Geometry check sheet. Reference: the model listing, model coordinates, mm. Face numbers are marked on the shaded views. A direction names the side the tool comes from. Coordinates: 2 decimals unless noted, no trailing zeros. Answer in a Markdown table with one row per item. Add a question column.
1. Mould release check, pull along Y, two halves, no side actions. Record for the marked faces 1, 2, 3 and 4: pulls with the +Y half, pulls with the -Y half, needs draft (parallel to the pull), parting line crosses it, or undercut.
2. Scan lines: L1, parallel to Z at x = -14.5, y = -33; L2, parallel to Z at x = -7, y = -28; L3, parallel to Y at x = 25, z = 4. Record each from-to range of solid material in increasing order. Write a range as from..to.
3. Depth check by flat-ended pin: P1, Ø5, axis at x = 20.5, y = -3, coming from the -Z side; P2, Ø1, axis at y = -28, z = 58.5, coming from the +X side; P3, Ø10, axis at x = -0.5, z = 55.5, coming from the +Y side. Enter the tip coordinate at first touch or a pass-through.
4. Cross-section at A-A on y = -25. Give the number of separate pieces and of enclosed holes in the cut face, and give its area (3 significant figures).
5. Set-up check for the marked faces 5, 6 and 7: record each of +Z, -Z, +X, -X, +Y, -Y from which the full face is reachable in a straight line by a thin tool's end or side.
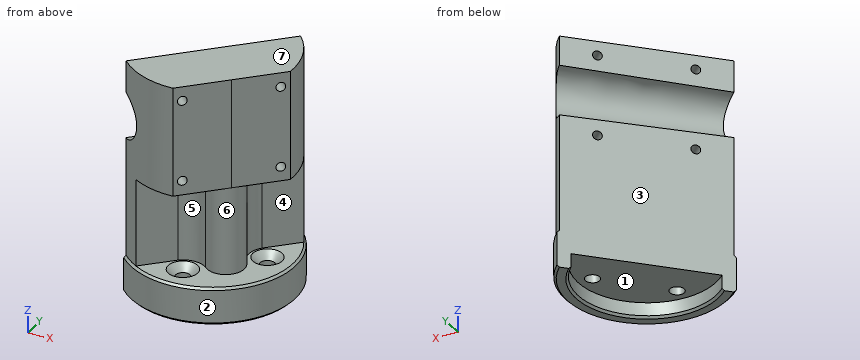
```python
from build123d import *

# Parameters (mm, degrees)
F1_ANGLE_BACK  = 45
F1_ANGLE       = 180
F2_SIZE        = 1
F4_D           = 6.6
F4_CSINK_D     = 13.44
F4_CSINK_ANGLE = 90
F6_DEPTH       = 40
F8_DEPTH       = 50
F12_D          = 4.1
F13_W          = 100.6186008453
F13_H          = 151.657152921
F14_DEPTH      = 0.5


# Not quite as in the source:
# - a feature names something its author has since deleted; it is built from what else it names


with BuildPart() as f1:
    # F0 (on Front) → F1 (revolve)
    with BuildSketch(Plane.XZ, mode=Mode.PRIVATE) as f1_sk:
        Polygon((0, 10), (0, 0), (31.6, 0), (31.6, -7), (37.5, -7), (37.5, 10), align=None)
    revolve(f1_sk.sketch.rotate(Axis((0, 0, 5), (0, 0, -1)), -F1_ANGLE_BACK), axis=Axis((0, 0, 5), (0, 0, -1)), revolution_arc=F1_ANGLE)

    # F2
    f2_edges = [f1.edges().sort_by_distance(p)[0] for p in [
        (22.344574, -22.344574, -7),
        (26.516504, -26.516504, -7),
        (26.516504, -26.516504, 10),
    ]]
    chamfer(f2_edges, length=F2_SIZE)

    # F4 (through all)
    with Locations(Plane.XY.offset(10)):
        with Locations((25, 0), (0, -25)):
            CounterSinkHole(F4_D / 2, F4_CSINK_D / 2, counter_sink_angle=F4_CSINK_ANGLE)

    # F5 (on face) → F6 (join)
    with BuildSketch(Plane.XY.offset(10)):
        with BuildLine():
            Line((19.4820004924, 5.3398648686), (7.0710678119, -7.0710678119))
            Line((7.0710678119, -7.0710678119), (-5.3398648686, -19.4820004924))
            ThreePointArc((-5.3398648686, -19.4820004924), (0.79408889, -17.1167209324), (7.0710678119, -19.0710678119))
            ThreePointArc((7.0710678119, -19.0710678119), (19.0710678119, -19.0710678119), (19.0710678119, -7.0710678119))
            ThreePointArc((19.0710678119, -7.0710678119), (17.1167209324, -0.79408889), (19.4820004924, 5.3398648686))
        make_face()
        with BuildLine():
            Line((7.0710678119, -7.0710678119), (0, 0))
            Line((0, 0), (-25.8093975133, -25.8093975133))
            ThreePointArc((-25.8093975133, -25.8093975133), (-21.9914756212, -29.1311688746), (-17.7507975491, -31.8929331729))
            Line((-17.7507975491, -31.8929331729), (-5.3398648686, -19.4820004924))
            Line((-5.3398648686, -19.4820004924), (7.0710678119, -7.0710678119))
        make_face()
        with BuildLine():
            Line((25.8093975133, 25.8093975133), (0, 0))
            Line((0, 0), (7.0710678119, -7.0710678119))
            Line((7.0710678119, -7.0710678119), (19.4820004924, 5.3398648686))
            Line((19.4820004924, 5.3398648686), (31.8929331729, 17.7507975491))
            ThreePointArc((31.8929331729, 17.7507975491), (29.1311688746, 21.9914756212), (25.8093975133, 25.8093975133))
        make_face()
    extrude(amount=F6_DEPTH)

    # F7 (on face) → F8 (join)
    with BuildSketch(Plane.XY.offset(50)):
        with BuildLine():
            ThreePointArc((36.4612769111, -1.6808587126), (35.531279534, 8.3533331479), (31.8929331729, 17.7507975491))
            Line((31.8929331729, 17.7507975491), (19.4820004924, 5.3398648686))
            ThreePointArc((19.4820004924, 5.3398648686), (17.1167209324, -0.79408889), (19.0710678119, -7.0710678119))
            ThreePointArc((19.0710678119, -7.0710678119), (21.5563491861, -13.0710678119), (19.0710678119, -19.0710678119))
            Line((19.0710678119, -19.0710678119), (36.4612769111, -1.6808587126))
        make_face()
        with BuildLine():
            Line((-5.3398648686, -19.4820004924), (-17.7507975491, -31.8929331729))
            ThreePointArc((-17.7507975491, -31.8929331729), (-8.3533331479, -35.531279534), (1.6808587126, -36.4612769111))
            Line((1.6808587126, -36.4612769111), (19.0710678119, -19.0710678119))
            ThreePointArc((19.0710678119, -19.0710678119), (13.0710678119, -21.5563491861), (7.0710678119, -19.0710678119))
            ThreePointArc((7.0710678119, -19.0710678119), (0.79408889, -17.1167209324), (-5.3398648686, -19.4820004924))
        make_face()
        with BuildLine():
            ThreePointArc((31.8929331729, 17.7507975491), (29.1311688746, 21.9914756212), (25.8093975133, 25.8093975133))
            Line((25.8093975133, 25.8093975133), (-25.8093975133, -25.8093975133))
            ThreePointArc((-25.8093975133, -25.8093975133), (-21.9914756212, -29.1311688746), (-17.7507975491, -31.8929331729))
            Line((-17.7507975491, -31.8929331729), (-5.3398648686, -19.4820004924))
            ThreePointArc((-5.3398648686, -19.4820004924), (0.79408889, -17.1167209324), (7.0710678119, -19.0710678119))
            ThreePointArc((7.0710678119, -19.0710678119), (13.0710678119, -21.5563491861), (19.0710678119, -19.0710678119))
            ThreePointArc((19.0710678119, -19.0710678119), (21.5563491861, -13.0710678119), (19.0710678119, -7.0710678119))
            ThreePointArc((19.0710678119, -7.0710678119), (17.1167209324, -0.79408889), (19.4820004924, 5.3398648686))
            Line((19.4820004924, 5.3398648686), (31.8929331729, 17.7507975491))
        make_face()
    extrude(amount=F8_DEPTH)

    # F9 (on face) → F10 (revolve, cut)
    with BuildSketch(Plane(origin=(0, 0, 0), x_dir=(-0.7071067812, -0.7071067812, 0), z_dir=(-0.7071067812, 0.7071067812, 0))):
        Polygon((36.5, 85.5), (-36.5, 86.5), (-36.5, 75), (36.5, 75), align=None)
    revolve(axis=Axis((0, 0, 75), (-0.7071067812, -0.7071067812, 0)), mode=Mode.SUBTRACT)

    # F12 (through all)
    with Locations(Plane(origin=(19.0710678119, -19.0710678119, 0), x_dir=(0.7071067812, 0.7071067812, 0), z_dir=(0.7071067812, -0.7071067812, 0))):
        with Locations((20.5934695606, 93.5), (20.5934695606, 56.5), (-20.5934695606, 56.5), (-20.5934695606, 93.5)):
            Hole(F12_D / 2)

    # F13 (on face) → F14 (cut)
    with BuildSketch(Plane(origin=(0, 0, 0), x_dir=(-0.7071067812, -0.7071067812, 0), z_dir=(-0.7071067812, 0.7071067812, 0))):
        with Locations((-1.9399225712, 37.7359148115)):
            Rectangle(F13_W, F13_H)
    extrude(amount=-F14_DEPTH, mode=Mode.SUBTRACT)


solid = f1.part
```
Results found:
| question | item | result |
|---|---|---|
| 1 | face 1 | undercut |
| 1 | face 2 | parting line crosses it |
| 1 | face 3 | pulls with the +Y half |
| 1 | face 4 | undercut |
| 2 | L1 | z = -7..10, 50..100 |
| 2 | L2 | z = 0..10, 50..100 |
| 2 | L3 | y = -27.95..-3.3, 3.3..24.29 |
| 3 | P1 | stops at z = 0 |
| 3 | P2 | stops at x = 10.64 |
| 3 | P3 | stops at y = 3.79 |
| 4 | separate pieces | 2 |
| 4 | enclosed holes | 2 |
| 4 | area | 2,670 mm^2 |
| 5 | face 5 | -Y |
| 5 | face 6 | none |
| 5 | face 7 | +Z, +X, -X, +Y, -Y |
